Autodesk Inventor part; units mm, degrees
ref_plane "Start Plane" through (0, 0, -57.0711) normal (0, 0, 1) x (1, 0, 0)
ref_plane "End Plane" through (0, 0, 2200) normal (0, 0, 1) x (1, 0, 0)
ref_plane "Work Plane4" through (60, 0, -60) normal (-0.7071, 0, -0.7071) x (-0.7071, 0, 0.7071)
ref_plane "Start Plane" through (0, 0, -57.0711) normal (0, 0, 1) x (1, 0, 0)
ref_plane "End Plane" through (0, 0, 2200) normal (0, 0, 1) x (1, 0, 0)
sketch "Sketch" plane through (0, 0, 0) normal (0, 0, 1) x (1, 0, 0)
  line L0 (-60, -50) -> (-60, 50)
  line L1 (-50, 60) -> (50, 60)
  line L2 (60, 50) -> (60, -50)
  line L3 (50, -60) -> (-50, -60)
  arc A0 (-60, -50) -> (-50, -60) centre (-50, -50) ccw
  arc A1 (60, 50) -> (50, 60) centre (50, 50) ccw
  arc A2 (-50, 60) -> (-60, 50) centre (-50, 50) ccw
  arc A3 (50, -60) -> (60, -50) centre (50, -50) ccw
  arc A4 (-50, 55) -> (-55, 50) centre (-50, 50) ccw
  line L4 (-50, 55) -> (50, 55)
  arc A5 (55, 50) -> (50, 55) centre (50, 50) ccw
  line L5 (55, 50) -> (55, -50)
  arc A6 (50, -55) -> (55, -50) centre (50, -50) ccw
  line L6 (50, -55) -> (-50, -55)
  arc A7 (-55, -50) -> (-50, -55) centre (-50, -50) ccw
  line L7 (-55, -50) -> (-55, 50)
  line L8 (0, 86.8995) -> (0, -86.8995) construction
  line L9 (-86.8995, 0) -> (86.8995, 0) construction
  dimension "d7" = 10
  dimension "d9" = 120
  dimension "d11" = 120
  dimension "d12" = 5
  dimension "d15" = 60
  dimension "d16" = 60
extrude "Body" add sketch "Sketch" along normal up to surface (2257.0711 mm away) from surface at -57.0711
sketch "Sketch3" plane through (0, 0, 0) normal (0, 0, 1) x (1, 0, 0)
  line L0 (0, 0) -> (10, 0)
ref_plane "Work Plane3" through (0, 0, 0) normal (0, -1, 0) x (1, 0, 0)
ref_plane "Work Plane4" through (60, 0, -60) normal (-0.7071, 0, -0.7071) x (-0.7071, 0, 0.7071)
split "Split1" plane through (60, 0, -60) removes the side toward (-0.7071, 0, -0.7071)
ref_plane "Work Plane5" through (0, -60, -60) normal (0, 0.7071, -0.7071) x (1, 0, 0)
split "Split2" plane through (0, -60, -60) removes the side toward (0, 0.7071, -0.7071)
sketch "Sketch4" plane through (0, 0, 0) normal (0, -1, 0) x (1, 0, 0)
  line L0 (-2, -57.0711) -> (12, -57.0711)
  line L1 (-2, 2200) -> (12, 2200)
  dimension "d18" = 2257.0711
equation "\"d7\" = G_IR"
equation "\"d9\" = G_W"
equation "\"d11\" = G_H"
equation "\"d12\" = G_T"
equation "\"d15\" = 0.5 * d9"
equation "\"d16\" = 0.5 * d11"
equation "\"d3\" = G_L"
equation "\"G_W\" = 120"
equation "\"G_H\" = 120"
equation "\"G_T\" = 5"
equation "\"G_IR\" = 10"
equation "\"G_L\" = d18"
equation "\"G_OFFSET_START\" = 57.07107"
equation "\"G_OFFSET_END\" = 0"
equation "\"d13\" = -G_OFFSET_START"
properties part number "ISO 10799-2 - 120x120x5 - 2257,07" material "Steel, Mild"
Input: part model. Units: mm. Frame: model coordinates. A direction names the side the tool comes from. Give positions to 0.01 mm unless a question says otherwise; leave off trailing zeros. Write each loop counter-clockwise with the first axis right and the second up, starting at its lowest first coordinate (ties: lowest second). Pieces come first, ordered by that corner, then holes. Notation, with made-up numbers: (-31, 25.5) - (22, 25.5) arc R14 ccw to (22, 39.5) - close; hole circle Ø10 at (15, -37.75). An arc over 180 degrees is marked (long way). Write item = value, one per line. Start each with the question number.
1) Draft query along Y for faces 3 (the face through (60, 1, 1059)), 4 (the face through (-1, 55, 1112)), 5 (the face through (-1, 60, 1115)). Return one class per face: pulls with the +Y half, pulls with the -Y half, needs draft (parallel to the pull), parting line crosses it, or undercut.
2) Cut plane C-C (z = 556.5). Return loops of the section in (x, y), and give its area (3 significant figures).
3) Reachability of faces 1 (the face through (55, 1, 1059)), 2 (the face through (1, -60, 1059)) from +Z, -Z, +X, -X, +Y, -Y: full face, straight path, thin tool, end or side. Return the list, or none.
4) Material intervals for L1, parallel to Y at x = 2.5, z = 483; L2, parallel to X at y = -54.5, z = 650.5, sorted ascending. Write a range as [from, to].
5) Cut plane B-B (y = 12). Return loops of the section in (x, z), and give its area (3 significant figures).
6) Cut plane A-A (x = -7). Return loops of the section in (y, z).
Answers follow:
q1.face_3 = needs draft
q1.face_4 = undercut
q1.face_5 = pulls with the +Y half
q2.outline = (-60, -50) arc R10 ccw to (-50, -60) - (50, -60) arc R10 ccw to (60, -50) - (60, 50) arc R10 ccw to (50, 60) - (-50, 60) arc R10 ccw to (-60, 50) - close; hole (-55, -50) arc R5 ccw to (-50, -55) - (50, -55) arc R5 ccw to (55, -50) - (55, 50) arc R5 ccw to (50, 55) - (-50, 55) arc R5 ccw to (-55, 50) - close
q2.area = 2,240 mm^2
q3.face_1 = +Z, -Z
q3.face_2 = +Z, -Z, +X, -X, -Y
q4.L1 = [-60, -55], [55, 60]
q4.L2 = [-58.93, -52.18], [52.18, 58.93]
q5.outline = (-60, 60) - (-55, 55) - (-55, 2200) - (-60, 2200) - close; (55, 12) - (60, 12) - (60, 2200) - (55, 2200) - close
q5.area = 21,700 mm^2
q6.outline = (-60, 7) - (-55, 7) - (-55, 2200) - (-60, 2200) - close; (55, 55) - (60, 60) - (60, 2200) - (55, 2200) - close
